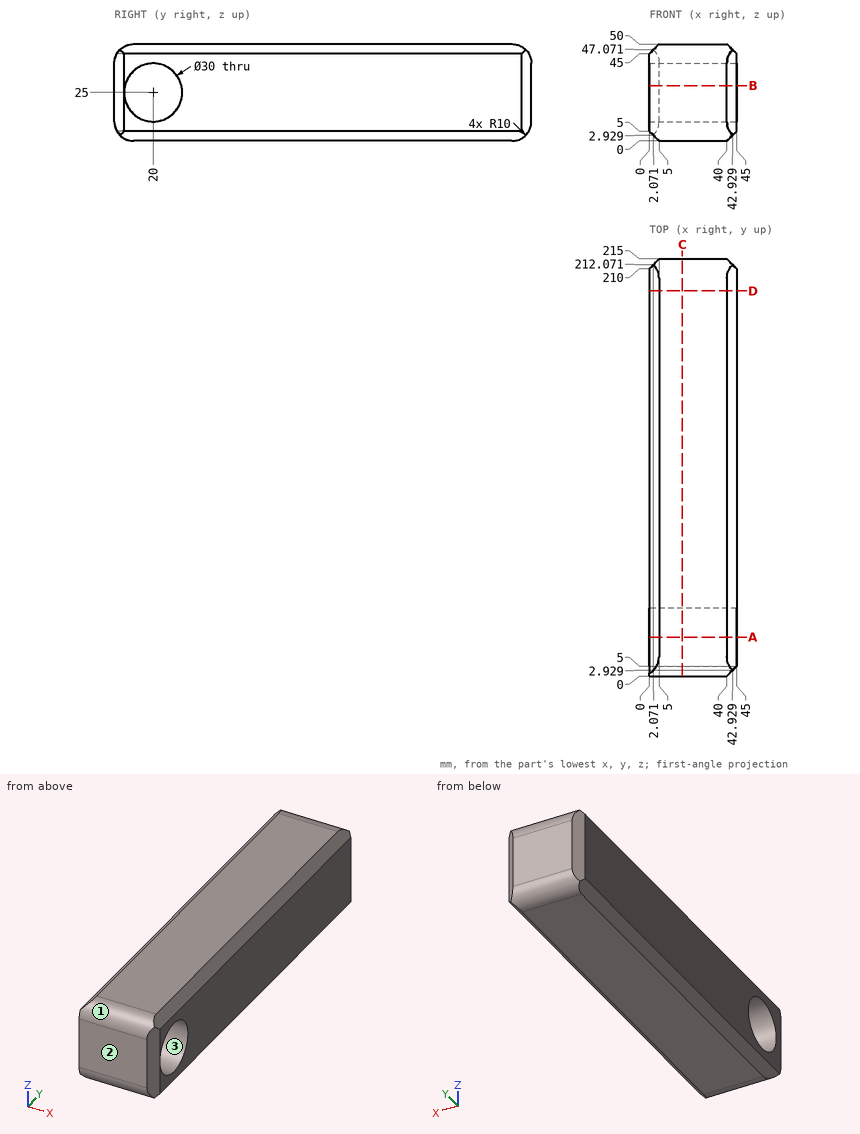
Design review of the part shown in the three views and the two pictorial views. Dimensions are in mm from the part's minimum x, y and z. Round coordinates to 2 decimals unless told otherwise and drop trailing zeros. Loops run counter-clockwise (first coordinate to the right, second up) from the corner with the lowest first, then second, coordinate; pieces in that order, holes last. Notation, with made-up numbers: (42.25, -38.5) - (90.25, -38.5) arc R35 cw to (90.25, -1.5) - close; hole circle Ø8 at (-33, -2.5). An arc over 180 degrees is marked (long way). Write each question's results on one line, items separated by ' | '. Start each with the question number.
Q1. Take a section at A-A on y = 20. Give the boundary of the cut face in (x, z).
Q2. Take a section at D-D on y = 198.5. Give the boundary of the cut face in (x, z), plus the area to 3 significant figures.
Q3. Take a section at C-C on x = 17. Give the boundary of the cut face in (y, z).
Q4. Take a section at B-B on z = 28.5. Give the boundary of the cut face in (x, y).
Q5. Draft analysis for pull direction Z (two halves, no side actions). For the marked faces 1, 2 and 3, state which applies: pulls with the +Z half, pulls with the -Z half, needs draft (parallel to the pull), parting line crosses it, or undercut.
Q6. Wall thickness on line 1 along Z through (x, y) = (19, 20); line 2 along Y through (x, z) = (27.5, 25); line 3 along Y through (x, z) = (22, 19.5): over which ranges is each line inside the solid? List them lowest first. Write a range as [from, to].
Q7. Insertion check: P1, Ø24, axis at y = 20, z = 25, coming from the +X side. The pin has a flat end and moves straight along its axis. Give the tip position at first contact, or say it passes through.
Data:
1) outline: (0, 5) - (5, 0) - (40, 0) - (45, 5) - (45, 10) - (0, 10) - close; (0, 40) - (45, 40) - (45, 45) - (40, 50) - (5, 50) - (0, 45) - close
2) outline: (0, 5) - (5, 0) - (40, 0) - (45, 5) - (45, 45) - (40, 50) - (5, 50) - (0, 45) - close | area: 2,200 mm²
3) outline: (0, 10) arc R10 ccw to (10, 0) - (205, 0) arc R10 ccw to (215, 10) - (215, 40) arc R10 ccw to (205, 50) - (10, 50) arc R10 ccw to (0, 40) - close; hole circle Ø30 at (20, 25)
4) outline: (0, 0) - (40, 0) - (45, 5) - (45, 5.41) - (0, 5.41) - close; (0, 34.59) - (45, 34.59) - (45, 210) - (40, 215) - (5, 215) - (0, 210) - close
5) face 1: pulls with the +Z half | face 2: needs draft | face 3: undercut
6) line 1: z = [0, 10], [40, 50] | line 2: y = [0, 5], [35, 215] | line 3: y = [0, 6.04], [33.96, 215]
7) P1: passes through
